Check sheet for the modelled part. Datum: model origin and axes. Units: mm. A direction names the side the tool comes from. Give positions to 0.01 mm unless a question says otherwise; leave off trailing zeros. Order: outer loops, then holes, each group sorted by start corner. A loop starts at its lowest first (then second) coordinate and runs counter-clockwise, first axis right, second up.
```python
from build123d import *

# Parameters (mm, degrees)
ESQUISSE1_R      = 19
ESQUISSE1_R_2    = 6
ESQUISSE1_R_3    = 2.5
EXTRUSION1_DEPTH = 7
ESQUISSE2_R      = 4.25
EXTRUSION2_DEPTH = 5


with BuildPart() as part:
    # Esquisse1 → Extrusion1 (new body)
    with BuildSketch(Plane.XY):
        Circle(ESQUISSE1_R)
        Circle(ESQUISSE1_R_2, mode=Mode.SUBTRACT)
        with Locations((12.340862004, -7.125)):
            Circle(ESQUISSE1_R_3, mode=Mode.SUBTRACT)
        with Locations((0, 14.25)):
            Circle(ESQUISSE1_R_3, mode=Mode.SUBTRACT)
        with Locations((-12.340862004, -7.125)):
            Circle(ESQUISSE1_R_3, mode=Mode.SUBTRACT)
    extrude(amount=EXTRUSION1_DEPTH)

    # Esquisse2 → Extrusion2 (cut)
    with BuildSketch(Plane.XY.offset(7)):
        with Locations((0, 14.25)):
            Circle(ESQUISSE2_R)
        with Locations((-12.340862004, -7.125)):
            Circle(ESQUISSE2_R)
        with Locations((12.340862004, -7.125)):
            Circle(ESQUISSE2_R)
    extrude(amount=-EXTRUSION2_DEPTH, mode=Mode.SUBTRACT)


solid = part.part
```
(1) Cross-section at D-D on z = 4.25. Enter the section's corners in (x, y) (3 decimals), then the cut area to 3 significant figures.
Response values:
outline: circle Ø38 at (0, 0); hole circle Ø8.5 at (-12.341, -7.125); hole circle Ø12 at (0, 0); hole circle Ø8.5 at (0, 14.25); hole circle Ø8.5 at (12.341, -7.125)
area: 851 mm2
(2) Cross-section at B-B on x = 0. Enter the section's corners in (y, z), then the cut area to 4 significant figures.
Response values:
outline: (-19, 0) - (-6, 0) - (-6, 7) - (-19, 7) - close; (6, 0) - (11.75, 0) - (11.75, 2) - (10, 2) - (10, 7) - (6, 7) - close; (16.75, 0) - (19, 0) - (19, 7) - (18.5, 7) - (18.5, 2) - (16.75, 2) - close
area: 129.5 mm2
(3) Cross-section at C-C on x = -11.5. Enter the section's corners in (y, z).
Response values:
outline: (-15.12, 0) - (-9.48, 0) - (-9.48, 2) - (-11.29, 2) - (-11.29, 7) - (-15.12, 7) - close; (-4.77, 0) - (15.12, 0) - (15.12, 7) - (-2.96, 7) - (-2.96, 2) - (-4.77, 2) - close
(4) Material ranges on L1, parallel to Y at x = 2, z = 4.75; L2, parallel to Z at x = 9.5, y = -6; L3, parallel to Y at x = 15.5, z = 6, recorded low to high.
Response values:
L1: y = -18.89 to -5.66, 5.66 to 10.5, 18 to 18.89
L2: z = 0 to 2
L3: y = -10.99 to -9.97, -4.28 to 10.99
(5) Cross-section at A-A on y = 0. Enter the section's corners in (x, z), then the cut area to 3 significant figures.
Response values:
outline: (-19, 0) - (-6, 0) - (-6, 7) - (-19, 7) - close; (6, 0) - (19, 0) - (19, 7) - (6, 7) - close
area: 182 mm2
(6) Gauge pin test, flat ends, axial feed: pin 1 Ø1.5 at (x, y) = (12, -8.5) entering from +Z; pin 2 Ø6 at (x, y) = (12.34, -7.12) entering from +Z; pin 3 Ø2 at (x, z) = (6.5, 1.5) entering from -Y; pin 4 Ø1 at (y, z) = (5.5, 3.5) entering from +X. Record the tip position at first contact, or that the pin passes through.
Response values:
pin 1: passes through
pin 2: stops at z = 2
pin 3: stops at y = -18.19
pin 4: stops at x = 18.33
(7) Set-up check for faces 1 (the face through (2, 12, 2)), 2 (the face through (-4.5, 4.5, 7)): record each of +Z, -Z, +X, -X, +Y, -Y from which the full face is reachable in a straight line by a thin tool's end or side.
Response values:
face 1: +Z
face 2: +Z, +X, -X, +Y, -Y
(8) Release check for a two-part mould opening along X. For faces 3 (the face through (-0.5, 11.8, 1)), 4 (the face through (-4.5, 4.5, 0)), 5 (the face through (8.767, -16.856, 3.451)) record: released by +X, released by -X, zero draft, split by the parting line, or undercut.
Response values:
face 3: undercut
face 4: zero draft
face 5: split by the parting line
